```python
from build123d import *

# Parameters (mm, degrees)
SKETCH_1_R      = 2
SKETCH_1_R_2    = 10
SKETCH_1_R_3    = 4
EXTRUDE_1_DEPTH = 3


with BuildPart() as part:
    # 草图1 → 凸台-拉伸1 (new body)
    with BuildSketch(Plane(origin=(0, 0, 0), x_dir=(1, 0, 0), z_dir=(0, 1, 0))):
        with BuildLine():
            Line((-78.915, 77.83), (-78.915, -77.83))
            ThreePointArc((-78.915, -77.83), (-75.986067812, -84.901067812), (-68.915, -87.83))
            Line((-68.915, -87.83), (68.915, -87.83))
            ThreePointArc((68.915, -87.83), (75.986067812, -84.901067812), (78.915, -77.83))
            Line((78.915, -77.83), (78.915, 77.83))
            ThreePointArc((78.915, 77.83), (75.986067812, 84.901067812), (68.915, 87.83))
            Line((68.915, 87.83), (-68.915, 87.83))
            ThreePointArc((-68.915, 87.83), (-75.986067812, 84.901067812), (-78.915, 77.83))
        make_face()
        with Locations(Location((72.465, 81.57, 0), (0, 0, 270))):
            Circle(SKETCH_1_R, mode=Mode.SUBTRACT)
        with Locations(Location((72.465, -81.57, 0), (0, 0, 90))):
            Circle(SKETCH_1_R, mode=Mode.SUBTRACT)
        with Locations(Location((-22.465, -81.57, 0), (0, 0, 270))):
            Circle(SKETCH_1_R, mode=Mode.SUBTRACT)
        with Locations(Location((-22.465, 81.57, 0), (0, 0, 90))):
            Circle(SKETCH_1_R, mode=Mode.SUBTRACT)
        with Locations(Location((-68.915, 77.83, 0), (0, 0, 270))):
            Circle(SKETCH_1_R, mode=Mode.SUBTRACT)
        with Locations(Location((-68.915, -77.83, 0), (0, 0, 90))):
            Circle(SKETCH_1_R, mode=Mode.SUBTRACT)
        with Locations(Location((25, 40, 0), (0, 0, 270))):
            Circle(SKETCH_1_R_2, mode=Mode.SUBTRACT)
        with Locations(Location((38.610158608, 53.633692132, 0), (0, 0, 90))):
            Circle(SKETCH_1_R, mode=Mode.SUBTRACT)
        with Locations(Location((38.610158608, 25.633692132, 0), (0, 0, 270))):
            Circle(SKETCH_1_R, mode=Mode.SUBTRACT)
        with Locations(Location((11.144228788, 25.633692132, 0), (0, 0, 90))):
            Circle(SKETCH_1_R, mode=Mode.SUBTRACT)
        with Locations(Location((25, -40, 0), (0, 0, 90))):
            Circle(SKETCH_1_R_2, mode=Mode.SUBTRACT)
        with Locations(Location((11.144228788, -25.633692132, 0), (0, 0, 270))):
            Circle(SKETCH_1_R, mode=Mode.SUBTRACT)
        with Locations(Location((38.610158608, -25.633692132, 0), (0, 0, 90))):
            Circle(SKETCH_1_R, mode=Mode.SUBTRACT)
        with Locations(Location((38.610158608, -53.633692132, 0), (0, 0, 270))):
            Circle(SKETCH_1_R, mode=Mode.SUBTRACT)
        with Locations(Location((11.144228788, -53.633692132, 0), (0, 0, 90))):
            Circle(SKETCH_1_R, mode=Mode.SUBTRACT)
        with Locations(Location((11.389841392, 53.633692132, 0), (0, 0, 270))):
            Circle(SKETCH_1_R, mode=Mode.SUBTRACT)
        with Locations(Location((63.82629955, 0, 0), (0, 0, 270))):
            Circle(SKETCH_1_R, mode=Mode.SUBTRACT)
        with Locations(Location((-13.82629955, 0, 0), (0, 0, 90))):
            Circle(SKETCH_1_R, mode=Mode.SUBTRACT)
        with Locations(Location((-3.290231438, 0, 0), (0, 0, 270))):
            Circle(SKETCH_1_R_3, mode=Mode.SUBTRACT)
    extrude(amount=EXTRUDE_1_DEPTH)


solid = part.part
```
Part model, mm, in its own coordinate system. Coordinates: 2 decimals unless noted, no trailing zeros. Order: outer loops, then holes, each group sorted by start corner. A loop starts at its lowest first (then second) coordinate and runs counter-clockwise, first axis right, second up. Notation, with made-up numbers: (-0.75, 51.25) - (6.25, 51.25) arc R9 ccw to (6.25, 63.25) - close; hole circle Ø4 at (24, -18.5). An arc over 180 degrees is marked (long way). Return JSON: item names as keys, results as strings. Group by question number.
Item 1: Pull direction X, two halves, no side cores. Call faces 1 (the face through (-70.6, 1.48, 76.75)), 2 (the face through (-76.063, 1.479, 84.823)), 3 (the face through (-19, 0, -1)): pulls with the +X half, pulls with the -X half, needs draft (parallel to the pull), parting line crosses it, or undercut.
Item 2: Cut at A-A (z = 40). List the corners of the cut face in (x, y) (3 decimals), plus the area to 3 significant figures.
Item 3: Pin check, flat tip, straight feed: pin 1 (2.5 mm diameter, centred on x = -68.915, z = 77.83, fed in from -Y). Stop position of the tip, or through.
Item 4: Cut at B-B (z = 0). List the corners of the cut face in (x, y) (3 decimals), plus the area to 3 significant figures.
Item 5: Cut at C-C (y = 2.35). State how many separate pieces and enclosed holes the cut face has, plus the area to 3 significant figures.
Item 6: Drill centre lines: probe 1 along X at (y, z) = (2.3, -81.57) (3 decimals); probe 2 along Z at (x, y) = (-23.5, 2.45); probe 3 along Z at (x, y) = (16.5, 0.55). Where is each one in solid material? Low to high. Write a range as from..to.
Check values:
{
 "1": {"face 1": "undercut", "face 2": "pulls with the -X half", "face 3": "needs draft"},
 "2": {"outline": "(-78.915, 0) - (15, 0) - (15, 3) - (-78.915, 3) - close; (35, 0) - (78.915, 0) - (78.915, 3) - (35, 3) - close", "area": "413 mm2"},
 "3": {"pin 1": "passes through"},
 "4": {"outline": "(-78.915, 0) - (-15.826, 0) - (-15.826, 3) - (-78.915, 3) - close; (-11.826, 0) - (-7.29, 0) - (-7.29, 3) - (-11.826, 3) - close; (0.71, 0) - (61.826, 0) - (61.826, 3) - (0.71, 3) - close; (65.826, 0) - (78.915, 0) - (78.915, 3) - (65.826, 3) - close", "area": "425 mm2"},
 "5": {"separate pieces": "1", "enclosed holes": "19", "area": "26,800 mm2"},
 "6": {"probe 1": "x = -78.189..-24.465, -20.465..70.465, 74.465..78.189", "probe 2": "z = -87.83..-83.28, -79.86..79.86, 83.28..87.83", "probe 3": "z = -87.83..-45.27, -34.73..34.73, 45.27..87.83"}
}
